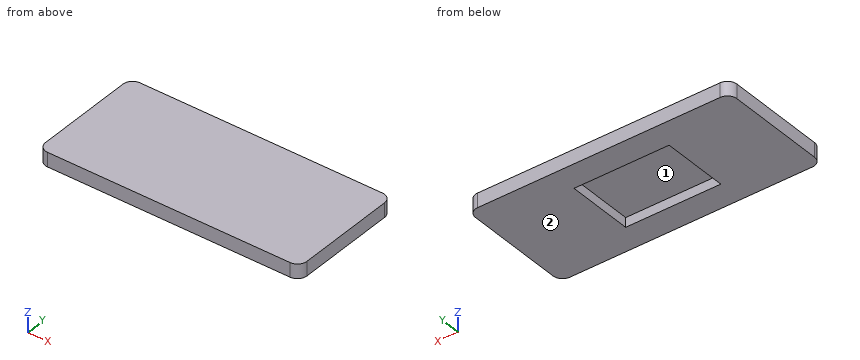
```python
from build123d import *

# Parameters (mm, degrees)
BOX001_W     = 20
BOX001_H     = 14
BOX001_DEPTH = 2
BOX_W        = 55
BOX_H        = 25
BOX_DEPTH    = 3
FILLET_R     = 2


with BuildPart() as cube001:
    # Box001 → Box001 (new body)
    with BuildSketch(Plane(origin=(6, -8, -3), x_dir=(1, 0, 0), z_dir=(0, 0, 1))):
        with Locations((10, 7)):
            Rectangle(BOX001_W, BOX001_H)
    extrude(amount=BOX001_DEPTH)


with BuildPart() as cut:
    # Box → Box (new body)
    with BuildSketch(Plane(origin=(-11, -13.5, -3), x_dir=(1, 0, 0), z_dir=(0, 0, 1))):
        with Locations((27.5, 12.5)):
            Rectangle(BOX_W, BOX_H)
    extrude(amount=BOX_DEPTH)

    # Fillet
    fillet_edges = [cut.edges().sort_by_distance(p)[0] for p in [
        (-11, -13.5, -1.5),
        (-11, 11.5, -1.5),
        (44, -13.5, -1.5),
        (44, 11.5, -1.5),
    ]]
    fillet(fillet_edges, radius=FILLET_R)

    # Cut: cut Cube001
    add(cube001.part, mode=Mode.SUBTRACT)


solid = cut.part
```
CAD build for the part. Positions are in the model's coordinates, mm. Face numbers are marked on the shaded views. Coordinates: 2 decimals unless noted, no trailing zeros. Loops run counter-clockwise (first coordinate to the right, second up) from the corner with the lowest first, then second, coordinate; pieces in that order, holes last. Notation, with made-up numbers: (78, 82) - (99, 82) arc R18 ccw to (99, 94) - close; hole circle Ø7 at (-31, 1). An arc over 180 degrees is marked (long way). Return JSON: item names as keys, results as strings.
1. Band-saw the part on C-C (x = 18.5). Give the cut face in (y, z), and give its area (3 significant figures).
Result:
{"outline": "(-13.5, -3) - (-8, -3) - (-8, -1) - (6, -1) - (6, -3) - (11.5, -3) - (11.5, 0) - (-13.5, 0) - close", "area": "47.0 mm2"}
2. Mould opens along Y. For the marked faces 1 and 2 say: released by +Y, released by -Y, zero draft, split by the parting line, or undercut.
Result:
{"face 1": "undercut", "face 2": "zero draft"}
3. Band-saw the part on A-A (z = -2.2). Give the cut face in (x, y).
Result:
{"outline": "(-11, -11.5) arc R2 ccw to (-9, -13.5) - (42, -13.5) arc R2 ccw to (44, -11.5) - (44, 9.5) arc R2 ccw to (42, 11.5) - (-9, 11.5) arc R2 ccw to (-11, 9.5) - close; hole (6, -8) - (26, -8) - (26, 6) - (6, 6) - close"}
4. Band-saw the part on B-B (y = -6.25). Give the cut face in (x, z), and give its area (3 significant figures).
Result:
{"outline": "(-11, -3) - (6, -3) - (6, -1) - (26, -1) - (26, -3) - (44, -3) - (44, 0) - (-11, 0) - close", "area": "125 mm2"}
5. Probe L1, parallel to X at y = 0.25, z = -2.3; L2, parallel to Y at x = 18.5, z = -1.6; L3, parallel to Z at x = 20, y = 5.75. List the from-to ranges inside material, lowest first. Write a range as from..to.
Result:
{"L1": "x = -11..6, 26..44", "L2": "y = -13.5..-8, 6..11.5", "L3": "z = -1..0"}
